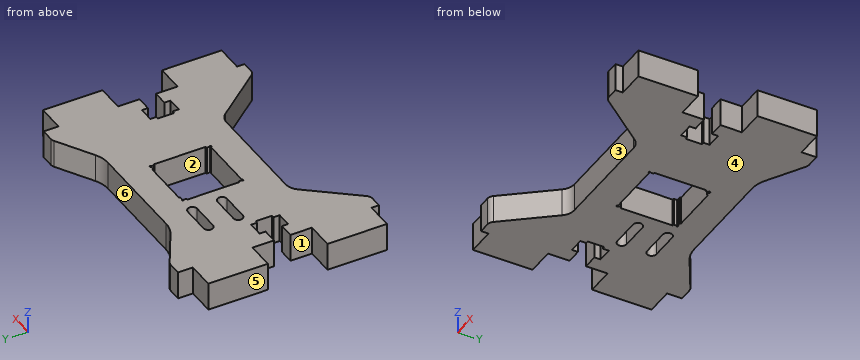
from build123d import *

# Parameters (mm, degrees)
SKETCH1_W           = 12.0904
SKETCH1_H           = 12.7
BOSS_EXTRUDE1_DEPTH = 5.969
CUT_EXTRUDE1_DEPTH  = 41.194496828
SKETCH3_R           = 0.1984375
CUT_EXTRUDE2_DEPTH  = 41.194496828
FILLET1_R           = 3.175
FILLET2_R           = 1.5875
SKETCH4_W           = 12.7
SKETCH4_H           = 11.1125
CUT_EXTRUDE3_DEPTH  = 41.194496828
FILLET7_R           = 0.1
SKETCH5_W           = 10.16
SKETCH5_H           = 0.5
CUT_EXTRUDE4_DEPTH  = 41.194496828
FILLET8_R           = 0.1
CUT_EXTRUDE5_DEPTH  = 41.194496828
FILLET9_R           = 6.35


with BuildPart() as part:
    # Sketch1 → Boss-Extrude1 (new body)
    with BuildSketch(Plane.XY):
        Polygon((25.4, 2.413), (25.4, -10.287), (31.242, -10.287), (31.242, -22.987), (25.4, -22.987), (25.4, -24.5745), (22.225, -24.5745), (12.7, -12.7), (-12.7, -12.7), (-22.225, -24.5745), (-25.4, -24.5745), (-25.4, -22.987), (-31.242, -22.987), (-31.242, -10.287), (-25.4, -10.287), (-25.4, 2.413), (-31.242, 2.413), (-31.242, 15.113), (-25.4, 15.113), (-25.4, 18.288), (-22.225, 18.288), (-12.7, 12.7), (12.7, 12.7), (22.225, 18.288), (25.4, 18.288), (25.4, 15.113), (31.242, 15.113), (31.242, 2.413), align=None)
        Rectangle(SKETCH1_W, SKETCH1_H, mode=Mode.SUBTRACT)
    extrude(amount=BOSS_EXTRUDE1_DEPTH)

    # Sketch2 → Cut-Extrude1 (cut, through all)
    with BuildSketch(Plane.XY.offset(5.969)):
        Polygon((22.225, -2.1844), (22.225, -0.889), (19.05, -0.889), (19.05, -2.1844), (18.492, -2.1844), (18.492, -5.6896), (19.05, -5.6896), (19.05, -6.985), (22.225, -6.985), (22.225, -5.6896), (25.4, -5.6896), (25.4, -2.1844), align=None)
        Polygon((-19.05, -2.1844), (-19.05, -0.889), (-22.225, -0.889), (-22.225, -2.1844), (-25.4, -2.1844), (-25.4, -5.6896), (-22.225, -5.6896), (-22.225, -6.985), (-19.05, -6.985), (-19.05, -5.6896), (-18.492, -5.6896), (-18.492, -2.1844), align=None)
    extrude(amount=-CUT_EXTRUDE1_DEPTH, mode=Mode.SUBTRACT)

    # Sketch3 → Cut-Extrude2 (cut, through all)
    with BuildSketch(Plane.XY.offset(5.969)):
        with Locations((6.0452, 6.35)):
            Circle(SKETCH3_R)
        with Locations((-6.0452, 6.35)):
            Circle(SKETCH3_R)
        with Locations((-6.0452, -6.35)):
            Circle(SKETCH3_R)
        with Locations((6.0452, -6.35)):
            Circle(SKETCH3_R)
    extrude(amount=-CUT_EXTRUDE2_DEPTH, mode=Mode.SUBTRACT)

    # Fillet1
    fillet1_edges = [part.edges().sort_by_distance(p)[0] for p in [
        (12.7, -12.7, 2.9845),
        (-12.7, -12.7, 2.9845),
    ]]
    fillet(fillet1_edges, radius=FILLET1_R)

    # Fillet2
    fillet2_edges = [part.edges().sort_by_distance(p)[0] for p in [
        (22.225, -24.5745, 2.9845),
        (-22.225, -24.5745, 2.9845),
        (-22.225, 18.288, 2.9845),
        (22.225, 18.288, 2.9845),
    ]]
    fillet(fillet2_edges, radius=FILLET2_R)

    # Sketch4 → Cut-Extrude3 (cut, through all)
    with BuildSketch(Plane.XY.offset(5.969)):
        Rectangle(SKETCH4_W, SKETCH4_H)
    extrude(amount=-CUT_EXTRUDE3_DEPTH, mode=Mode.SUBTRACT)

    # Fillet7
    fillet7_edges = [part.edges().sort_by_distance(p)[0] for p in [
        (6.0452, -5.55625, 2.9845),
        (6.0452, 5.55625, 2.9845),
        (-6.0452, 5.55625, 2.9845),
        (-6.35, 5.55625, 2.9845),
        (-6.0452, -5.55625, 2.9845),
        (-6.35, -5.55625, 2.9845),
        (6.35, 5.55625, 2.9845),
        (6.35, -5.55625, 2.9845),
    ]]
    fillet(fillet7_edges, radius=FILLET7_R)

    # Sketch5 → Cut-Extrude4 (cut, through all)
    with BuildSketch(Plane.XY.offset(5.969)):
        with Locations((0, 6.35)):
            Rectangle(SKETCH5_W, SKETCH5_H)
    extrude(amount=-CUT_EXTRUDE4_DEPTH, mode=Mode.SUBTRACT)

    # Fillet8
    fillet8_edges = [part.edges().sort_by_distance(p)[0] for p in [
        (5.08, 6.35, 2.9845),
        (-5.08, 6.35, 2.9845),
        (-5.08, 6.6, 2.9845),
        (5.08, 6.6, 2.9845),
    ]]
    fillet(fillet8_edges, radius=FILLET8_R)

    # Sketch6 → Cut-Extrude5 (cut, through all)
    with BuildSketch(Plane.XY.offset(5.969)):
        with BuildLine():
            Line((-15.7, 7.35), (-9.7, 7.35))
            ThreePointArc((-9.7, 7.35), (-8.7, 6.35), (-9.7, 5.35))
            Line((-9.7, 5.35), (-15.7, 5.35))
            ThreePointArc((-15.7, 5.35), (-16.7, 6.35), (-15.7, 7.35))
        make_face()
        with BuildLine():
            Line((-15.7, 1), (-9.7, 1))
            ThreePointArc((-9.7, 1), (-8.7, 0), (-9.7, -1))
            Line((-9.7, -1), (-15.7, -1))
            ThreePointArc((-15.7, -1), (-16.7, 0), (-15.7, 1))
        make_face()
    extrude(amount=-CUT_EXTRUDE5_DEPTH, mode=Mode.SUBTRACT)

    # Fillet9
    fillet9_edges = [part.edges().sort_by_distance(p)[0] for p in [
        (-12.7, 12.7, 2.9845),
        (12.7, 12.7, 2.9845),
    ]]
    fillet(fillet9_edges, radius=FILLET9_R)


solid = part.part
Geometry check sheet. Reference: the model listing, model coordinates, mm. Face numbers are marked on the shaded views. A direction names the side the tool comes from. Give positions to 0.01 mm unless a question says otherwise; leave off trailing zeros. Loops run counter-clockwise (first coordinate to the right, second up) from the corner with the lowest first, then second, coordinate; pieces in that order, holes last.
(1) Release check for a two-part mould opening along X. For the marked faces 4, 5 and 6 record: released by +X, released by -X, zero draft, split by the parting line, or undercut.
From the geometry:
face 4: zero draft
face 5: released by -X
face 6: undercut
(2) Section check B-B on z = 0.8. Count the separate pieces of the cut face and the enclosed holes in it, then the cut area to 3 significant figures.
From the geometry:
separate pieces: 1
enclosed holes: 3
area: 1,610 mm2
(3) Section check A-A on x = 1.5. Record the cut outline in (y, z).
From the geometry:
outline: (-12.7, 0) - (-6.35, 0) - (-6.35, 5.97) - (-12.7, 5.97) - close; (6.6, 0) - (12.7, 0) - (12.7, 5.97) - (6.6, 5.97) - close
(4) Section check D-D on x = 15.5. Record the cut outline in (y, z).
From the geometry:
outline: (-16.19, 0) - (14.34, 0) - (14.34, 5.97) - (-16.19, 5.97) - close
(5) Set-up check for the marked faces 1, 2 and 3: record each of +Z, -Z, +X, -X, +Y, -Y from which the full face is reachable in a straight line by a thin tool's end or side.
From the geometry:
face 1: +Z, -Z, -X
face 2: +Z, -Z
face 3: +Z, -Z, -Y
(6) Section check C-C on x = -26.5. Record the cut outline in (y, z), then the cut area to 3 significant figures.
From the geometry:
outline: (-22.99, 0) - (-10.29, 0) - (-10.29, 5.97) - (-22.99, 5.97) - close; (2.41, 0) - (15.11, 0) - (15.11, 5.97) - (2.41, 5.97) - close
area: 152 mm2
(7) Depth check by flat-ended pin: pin 1 Ø3 at (x, z) = (1, 2.5) entering from +Y; pin 2 Ø1 at (x, z) = (-21, 3.5) entering from +Y; pin 3 Ø3 at (x, z) = (-11.5, 1.5) entering from +Y. Enter the tip coordinate at first touch or a pass-through.
From the geometry:
pin 1: stops at y = 12.7
pin 2: stops at y = 17.86
pin 3: stops at y = 13.03
(8) Thickness scan on L1, parallel to Y at x = -10, z = 3.7; L2, parallel to Y at x = -2, z = 1.95; L3, parallel to X at y = -5, z = 1.05. Record the ranges inside material, lowest first.
From the geometry:
L1: y = -12.7 to -1, 1 to 5.35, 7.35 to 12.7
L2: y = -12.7 to -6.35, 6.6 to 12.7
L3: x = -18.49 to -6.35, 6.35 to 18.49
